Answer from the drawing. Dimensions are ordinates in mm from the lowest x, y and z of the part. A direction names the side the tool comes from. Coordinates: 2 decimals unless noted, no trailing zeros. Write each loop counter-clockwise with the first axis right and the second up, starting at its lowest first coordinate (ties: lowest second). Pieces come first, ordered by that corner, then holes.
(1) Straight lines are drawn through the part: line 1 (X direction, y = 1119, z = 571); line 2 (Z direction, x = 381, y = 1085); line 3 (Y direction, x = 1905, z = 90). For each, find the intervals that lie inside material, in ascending order.
(2) Which of the six approach directions +Z, -Z, +X, -X, +Y, -Y give full straight-line access (tool end or side, diameter ignored) to the marked faces 1, 2 and 3?
(3) The part is cut by section B-B on x = 381. Determine the outline of the cut face in (y, z), plus the area to 3 significant figures.
(4) The part is cut by section A-A on z = 985.5. Determine the outline of the cut face in (x, y), plus the area to 3 significant figures.
(5) The part is cut by section C-C on y = 571.5. Determine the outline of the cut face in (x, z), plus the area to 3 significant figures.
(6) Given P1, Ø1.5, axis at x = 1110, z = 164, coming from the -Y side, flat-ended and moving along its own axis, determine where the tip first touches the part or whether it passes through.
(7) The part is cut by section D-D on z = 141.5. Determine the outline of the cut face in (x, y).
(8) For a pull along X with two mould halves and no side action, classify the marked faces 4, 5, 6 and 7 as +X half, -X half, draft (parallel to the pull), parting line (faces both ways), or undercut.
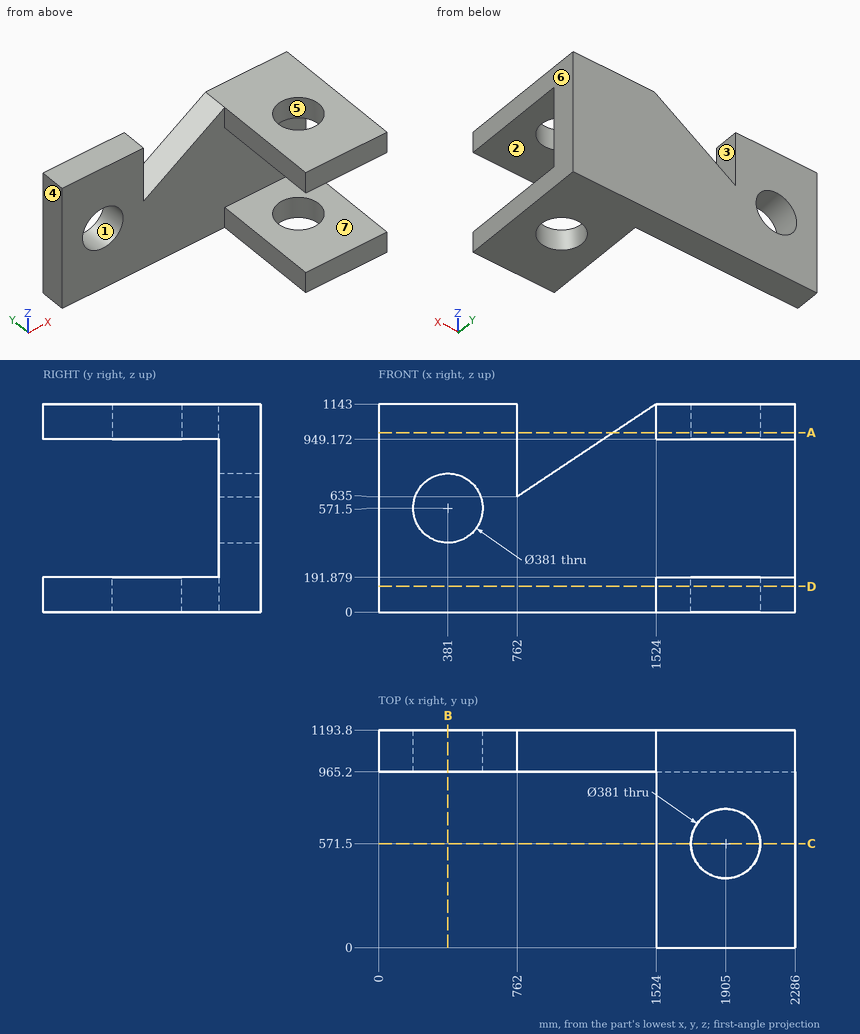
Model answer:
1. line 1: x = 0 to 190.5, 571.5 to 2286
1. line 2: z = 0 to 381, 762 to 1143
1. line 3: y = 0 to 381, 762 to 1193.8
2. face 1: +Y, -Y
2. face 2: +X, -X, -Y
2. face 3: +Z, +Y, -Y
3. outline: (965.2, 0) - (1193.8, 0) - (1193.8, 381) - (965.2, 381) - close; (965.2, 762) - (1193.8, 762) - (1193.8, 1143) - (965.2, 1143) - close
3. area: 174,000 mm2
4. outline: (0, 965.2) - (762, 965.2) - (762, 1193.8) - (0, 1193.8) - close; (1287.75, 965.2) - (1524, 965.2) - (1524, 0) - (2286, 0) - (2286, 1193.8) - (1287.75, 1193.8) - close; hole circle Ø381 at (1905, 571.5)
4. area: 1,020,000 mm2
5. outline: (1524, 0) - (1714.5, 0) - (1714.5, 191.88) - (1524, 191.88) - close; (1524, 949.17) - (1714.5, 949.17) - (1714.5, 1143) - (1524, 1143) - close; (2095.5, 0) - (2286, 0) - (2286, 191.88) - (2095.5, 191.88) - close; (2095.5, 949.17) - (2286, 949.17) - (2286, 1143) - (2095.5, 1143) - close
5. area: 147,000 mm2
6. P1: stops at y = 965.2
7. outline: (0, 965.2) - (1524, 965.2) - (1524, 0) - (2286, 0) - (2286, 1193.8) - (0, 1193.8) - close; hole circle Ø381 at (1905, 571.5)
8. face 4: -X half
8. face 5: undercut
8. face 6: +X half
8. face 7: draft
